from build123d import *

# Parameters (mm, degrees)
F1_DEPTH = 2.5
F0_W     = 1.443921
F0_H     = 0.75
F2_DEPTH = 1
F3_DEPTH = 0.3125
F0_W_2   = 0.551202
F0_H_2   = 1.125
F5_R     = 0.2


with BuildPart() as f1:
    # F0 (on Front) → F1 (new body, symmetric)
    with BuildSketch(Plane.XZ):
        Polygon((-1.625, -0.375), (1.625, -0.375), (1.625, 0.375), (0.875, 0.375), (-1.625, 0.375), align=None)
    extrude(amount=F1_DEPTH, both=True)

    # F0 (on Front) → F2 (join, symmetric)
    with BuildSketch(Plane.XZ):
        with BuildLine():
            Line((0.875, 0.375), (1.625, 0.375))
            Line((1.625, 0.375), (1.625, 1.063))
            ThreePointArc((1.625, 1.063), (1.808058, 1.504942), (2.25, 1.688))
            Line((2.25, 1.688), (2.375, 1.688))
            Line((2.375, 1.688), (2.375, 2.438))
            Line((2.375, 2.438), (2.25, 2.438))
            add(Edge.make_bspline(
                [(2.121971, 2.432026), (2.164984, 2.434706), (2.207675, 2.436705), (2.25, 2.438)],
                knots=[4.277425, 4.277425, 4.277425, 4.277425, 4.389942, 4.389942, 4.389942, 4.389942], degree=3))
            ThreePointArc((2.121971, 2.432026), (1.23347, 1.988901), (0.875, 1.063))
            Line((0.875, 1.063), (0.875, 0.375))
        make_face()
        with Locations((3.09696, 2.063)):
            Rectangle(F0_W, F0_H)
    extrude(amount=F2_DEPTH, both=True)

    # F0 (on Front) → F3 (join, symmetric)
    with BuildSketch(Plane.XZ):
        with BuildLine():
            add(Edge.make_bspline(
                [(-1.625, 0.375), (-1.612032, 1.243352), (0.486814, 2.330145), (2.121971, 2.432026)],
                knots=[0, 0, 0, 0, 4.277425, 4.277425, 4.277425, 4.277425], degree=3))
            Line((-1.625, 0.375), (0.875, 0.375))
            Line((0.875, 0.375), (0.875, 1.063))
            ThreePointArc((0.875, 1.063), (1.23347, 1.988901), (2.121971, 2.432026))
        make_face()
    extrude(amount=F3_DEPTH, both=True)

    # F0 (on Front) → F4 (revolve)
    with BuildSketch(Plane.XZ):
        with Locations((4.099399, 2.0625)):
            Rectangle(F0_W_2, F0_H_2)
    revolve(axis=Axis((3.823798, 0, 2.0625), (0, 0, 1)))

    # F5
    f5_edges = [f1.edges().sort_by_distance(p)[0] for p in [
        (-1.625, -2.5, 0),
        (1.625, -2.5, 0),
        (1.625, 2.5, 0),
        (-1.625, 2.5, 0),
    ]]
    fillet(f5_edges, radius=F5_R)


solid = f1.part
For this review, take the finished solid that the model builds, in its own axes (mm). A direction names the side the tool comes from. Give positions to 0.01 mm unless a question says otherwise; leave off trailing zeros. Order: outer loops, then holes, each group sorted by start corner. A loop starts at its lowest first (then second) coordinate and runs counter-clockwise, first axis right, second up. Notation, with made-up numbers: M 78,-19.75 L 90,-19.75 A36 ccw 90,19.25 Z; hole C -11.75,87.25 d3. An arc over 180 degrees is marked long. Answer in a Markdown table with one row per item. Add a question column.
(1) Consider section B-B on y = -1.45. State the section outline as (x, z) points (3 decimals), and give its area (3 significant figures).
(2) For faces 1 (the face through (4, 0, 1.5)), 2 (the face through (1.243, 0.651, 1.999)), 3 (the face through (1.243, -0.661, 1.999)), 4 (the face through (2, -1, 2)), 5 (the face through (2, 1, 2)), list the 3-axis set-ups (+Z, -Z, +X, -X, +Y, -Y) from which the entire face can be reached by the end or side of a thin tool; tool diameter is ignored.
(3) Wall thickness on probe 1 along Z at (x, y) = (0.75, 2.05) (3 decimals); probe 2 along Y at (x, z) = (1, 1.05); probe 3 along X at (y, z) = (0.4, 0.2) (3 decimals): over which ranges is each line inside the solid? List them lowest first. Write a range as [from, to].
(4) For pin 1 (1.8 mm diameter, centred on x = -0.5, y = 1.5, fed in from +Z) (3 decimals); pin 2 (0.5 mm diameter, centred on y = -1, z = 2, fed in from +X); pin 3 (1.5 mm diameter, centred on y = -2, z = 2, fed in from +X); pin 4 (0.6 mm diameter, centred on x = 0, z = 1, fed in from +Y), all flat-tipped, find the tip position at first contact; note any pin that passes through.
(5) Consider section C-C on x = 3. State the section outline as (y, z) points.
(6) Consider section A-A on z = -0.05. State the section outline as (x, y) points (3 decimals).
Evaluation:
| question | item | result |
|---|---|---|
| 1 | outline | M -1.625,-0.375 L 1.625,-0.375 L 1.625,0.375 L -1.625,0.375 Z |
| 1 | area | 2.44 mm^2 |
| 2 | face 1 | -Z, +X, +Y, -Y |
| 2 | face 2 | +Z, -X, +Y |
| 2 | face 3 | +Z, -X, -Y |
| 2 | face 4 | +Z, +X, -X, -Y |
| 2 | face 5 | +Z, +X, -X, +Y |
| 3 | probe 1 | z = [-0.375, 0.375] |
| 3 | probe 2 | y = [-1, 1] |
| 3 | probe 3 | x = [-1.625, 1.625] |
| 4 | pin 1 | stops at z = 0.375 |
| 4 | pin 2 | stops at x = 3.82 |
| 4 | pin 3 | passes through |
| 4 | pin 4 | stops at y = 0.31 |
| 5 | outline | M -1,1.69 L 1,1.69 L 1,2.44 L -1,2.44 Z |
| 6 | outline | M -1.625,-2.3 A0.2 ccw -1.425,-2.5 L 1.425,-2.5 A0.2 ccw 1.625,-2.3 L 1.625,2.3 A0.2 ccw 1.425,2.5 L -1.425,2.5 A0.2 ccw -1.625,2.3 Z |
